Input: part model. Units: mm. Frame: model coordinates. Face numbers are marked on the shaded views. Coordinates: 2 decimals unless noted, no trailing zeros. Order: outer loops, then holes, each group sorted by start corner. A loop starts at its lowest first (then second) coordinate and runs counter-clockwise, first axis right, second up. Notation, with made-up numbers: M 1.25,58.25 L 6.25,58.25 A23 cw 6.25,83.25 Z; hole C 60,11.25 d2. An arc over 180 degrees is marked long. Answer in a Markdown table with one row per item.
from build123d import *

# Parameters (mm, degrees)
CYLINDER006_R     = 1.25
CYLINDER006_DEPTH = 10
CYLINDER007_R     = 1.25
CYLINDER007_DEPTH = 10
CYLINDER008_R     = 1.25
CYLINDER008_DEPTH = 10
CYLINDER001_R     = 1.25
CYLINDER001_DEPTH = 10
CYLINDER003_R     = 1.1
CYLINDER003_DEPTH = 10
CYLINDER004_R     = 1.1
CYLINDER004_DEPTH = 10
CYLINDER005_R     = 1.1
CYLINDER005_DEPTH = 10
CYLINDER002_R     = 1.1
CYLINDER002_DEPTH = 10
CYLINDER_R        = 14
CYLINDER_DEPTH    = 10
BOX_W             = 44
BOX_H             = 32
BOX_DEPTH         = 5
CHAMFER_SIZE      = 1.5
CHAMFER001_SIZE   = 1.5


with BuildPart() as cylinder006:
    # Cylinder006 → Cylinder006 (new body)
    with BuildSketch(Plane(origin=(10, 28, 0), x_dir=(1, 0, 0), z_dir=(0, 0, 1))):
        Circle(CYLINDER006_R)
    extrude(amount=CYLINDER006_DEPTH)


with BuildPart() as cylinder007:
    # Cylinder007 → Cylinder007 (new body)
    with BuildSketch(Plane(origin=(34, 28, 0), x_dir=(1, 0, 0), z_dir=(0, 0, 1))):
        Circle(CYLINDER007_R)
    extrude(amount=CYLINDER007_DEPTH)


with BuildPart() as cylinder008:
    # Cylinder008 → Cylinder008 (new body)
    with BuildSketch(Plane(origin=(34, 4, 0), x_dir=(1, 0, 0), z_dir=(0, 0, 1))):
        Circle(CYLINDER008_R)
    extrude(amount=CYLINDER008_DEPTH)


with BuildPart() as fusion001:
    # Cylinder001 → Cylinder001 (new body)
    with BuildSketch(Plane(origin=(10, 4, 0), x_dir=(1, 0, 0), z_dir=(0, 0, 1))):
        Circle(CYLINDER001_R)
    extrude(amount=CYLINDER001_DEPTH)

    # Fusion001: union Cylinder006, Cylinder007, Cylinder008
    add(cylinder006.part)
    add(cylinder007.part)
    add(cylinder008.part)


with BuildPart() as cylinder003:
    # Cylinder003 → Cylinder003 (new body)
    with BuildSketch(Plane(origin=(3, 27.75, 0), x_dir=(1, 0, 0), z_dir=(0, 0, 1))):
        Circle(CYLINDER003_R)
    extrude(amount=CYLINDER003_DEPTH)


with BuildPart() as cylinder004:
    # Cylinder004 → Cylinder004 (new body)
    with BuildSketch(Plane(origin=(41, 4.25, 0), x_dir=(1, 0, 0), z_dir=(0, 0, 1))):
        Circle(CYLINDER004_R)
    extrude(amount=CYLINDER004_DEPTH)


with BuildPart() as cylinder005:
    # Cylinder005 → Cylinder005 (new body)
    with BuildSketch(Plane(origin=(41, 27.75, 0), x_dir=(1, 0, 0), z_dir=(0, 0, 1))):
        Circle(CYLINDER005_R)
    extrude(amount=CYLINDER005_DEPTH)


with BuildPart() as fusion:
    # Cylinder002 → Cylinder002 (new body)
    with BuildSketch(Plane(origin=(3, 4.25, 0), x_dir=(1, 0, 0), z_dir=(0, 0, 1))):
        Circle(CYLINDER002_R)
    extrude(amount=CYLINDER002_DEPTH)

    # Fusion: union Cylinder003, Cylinder004, Cylinder005
    add(cylinder003.part)
    add(cylinder004.part)
    add(cylinder005.part)


with BuildPart() as cylinder:
    # Cylinder → Cylinder (new body)
    with BuildSketch(Plane(origin=(22, 16, -1), x_dir=(1, 0, 0), z_dir=(0, 0, 1))):
        Circle(CYLINDER_R)
    extrude(amount=CYLINDER_DEPTH)


with BuildPart() as chamfer001:
    # Box → Box (new body)
    with BuildSketch(Plane.XY.offset(1)):
        with Locations((22, 16)):
            Rectangle(BOX_W, BOX_H)
    extrude(amount=BOX_DEPTH)

    # Cut: cut Cylinder
    add(cylinder.part, mode=Mode.SUBTRACT)

    # Cut001: cut Fusion
    add(fusion.part, mode=Mode.SUBTRACT)

    # Cut002: cut Fusion001
    add(fusion001.part, mode=Mode.SUBTRACT)

    # Chamfer
    chamfer_edges = [chamfer001.edges().sort_by_distance(p)[0] for p in [
        (8.75, 28, 6),
    ]]
    chamfer(chamfer_edges, length=CHAMFER_SIZE)

    # Chamfer001
    chamfer001_edges = [chamfer001.edges().sort_by_distance(p)[0] for p in [
        (32.75, 4, 6),
        (32.75, 28, 6),
        (8.75, 4, 6),
    ]]
    chamfer(chamfer001_edges, length=CHAMFER001_SIZE)


solid = chamfer001.part
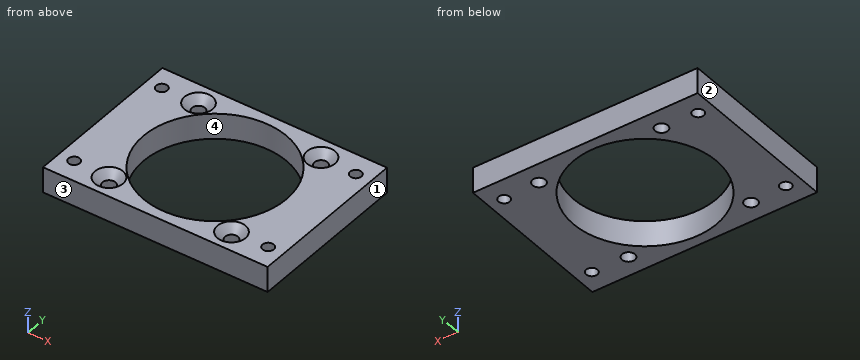
1) Cut plane A-A, the plane y = 16. Output: boundary loops of the cut face in (x, z), and give its area (3 significant figures).
Resolved:
| item | result |
|---|---|
| outline | M 0,1 L 8,1 L 8,6 L 0,6 Z; M 36,1 L 44,1 L 44,6 L 36,6 Z |
| area | 80.0 mm2 |
2) Cut plane B-B, the plane x = 41. Output: boundary loops of the cut face in (y, z).
Resolved:
| item | result |
|---|---|
| outline | M 0,1 L 3.15,1 L 3.15,6 L 0,6 Z; M 5.35,1 L 26.65,1 L 26.65,6 L 5.35,6 Z; M 28.85,1 L 32,1 L 32,6 L 28.85,6 Z |
3) Contact query for a flat-ended pin moving along its axis: pin 1 (4 mm diameter, centred on x = 10, y = 28, fed in from +Z). Output: stop coordinate, or through.
Resolved:
| item | result |
|---|---|
| pin 1 | stops at z = 5.25 |
4) Material intervals for probe 1 along Y at (x, z) = (41, 3.1); probe 2 along Y at (x, z) = (34, 3.3); probe 3 along X at (y, z) = (4.25, 3.3), sorted ascending.
Resolved:
| item | result |
|---|---|
| probe 1 | y = 0 to 3.15, 5.35 to 26.65, 28.85 to 32 |
| probe 2 | y = 0 to 2.75, 5.25 to 8.79, 23.21 to 26.75, 29.25 to 32 |
| probe 3 | x = 0 to 1.9, 4.1 to 8.78, 11.22 to 14.39, 29.61 to 32.78, 35.22 to 39.9, 42.1 to 44 |
5) Cut plane C-C, the plane z = 5.45. State how many separate pieces and enclosed holes the cut face has, and give its area (3 significant figures).
Resolved:
| item | result |
|---|---|
| separate pieces | 1 |
| enclosed holes | 9 |
| area | 716 mm2 |
6) Cut plane D-D, the plane x = 20.5. Output: boundary loops of the cut face in (y, z), and give its area (3 significant figures).
Resolved:
| item | result |
|---|---|
| outline | M 0,1 L 2.08,1 L 2.08,6 L 0,6 Z; M 29.92,1 L 32,1 L 32,6 L 29.92,6 Z |
| area | 20.8 mm2 |
7) Mould query, pull axis X, two halves, no side actions, for the marked faces 1, 2, 3 and 4. Classes: +X half, -X half, draft (parallel to the pull), parting line (faces both ways), or undercut.
Resolved:
| item | result |
|---|---|
| face 1 | +X half |
| face 2 | -X half |
| face 3 | draft |
| face 4 | undercut |
